from build123d import *
from OCP.BRepFilletAPI import BRepFilletAPI_MakeChamfer

# Parameters (mm, degrees)
SKETCH_1_W                = 265
SKETCH_1_H                = 125
EXTRUDE_1_DEPTH           = 85
SKETCH_2_W                = 330
SKETCH_2_H                = 125
EXTRUDE_2_DEPTH           = 20
SKETCH_3_W                = 150
SKETCH_3_H                = 125
CUT_EXTRUDE_1_DEPTH       = 5
SKETCH_4_R                = 40
CUT_EXTRUDE_2_DEPTH       = 206.319872394
SKETCH_5_W                = 210
SKETCH_5_H                = 125
CUT_EXTRUDE_3_DEPTH       = 80
CHAMFER_2_SIZE            = 56
CHAMFER_2_SIZE2           = 32.331615075
SKETCH_10_R               = 4.5
SKETCH_10_R_2             = 4
CUT_EXTRUDE_4_DEPTH       = 196.847517217
HOLE_WIZARD_M16_1_D       = 14
HOLE_WIZARD_M16_1_DEPTH   = 20
HOLE_WIZARD_M16_1_TIP     = 4.206024333
CHAMFER_3_SIZE            = 1
HOLE_WIZARD_1_D           = 9
HOLE_WIZARD_1_CBORE_D     = 15
HOLE_WIZARD_1_CBORE_DEPTH = 9
HOLE_WIZARD_M8_1_D        = 6.8
HOLE_WIZARD_M8_1_DEPTH    = 22.25
HOLE_WIZARD_M8_1_TIP      = 2.042926105
FILLET_1_R                = 8
FILLET_2_R                = 2


with BuildPart() as part:
    # 草图1 → 凸台-拉伸1 (new body)
    with BuildSketch(Plane.XY):
        Rectangle(SKETCH_1_W, SKETCH_1_H)
    extrude(amount=EXTRUDE_1_DEPTH)

    # 草图2 → 凸台-拉伸2 (add)
    with BuildSketch(Plane.XY.offset(85)):
        Rectangle(SKETCH_2_W, SKETCH_2_H)
    extrude(amount=EXTRUDE_2_DEPTH)

    # 草图3 → 切除-拉伸1 (cut)
    with BuildSketch(Plane(origin=(0, 0, 0), x_dir=(-1, 0, 0), z_dir=(0, 0, -1))):
        Rectangle(SKETCH_3_W, SKETCH_3_H)
    extrude(amount=-CUT_EXTRUDE_1_DEPTH, mode=Mode.SUBTRACT)

    # 草图4 → 切除-拉伸2 (cut, through all)
    with BuildSketch(Plane(origin=(0, 0, 0), x_dir=(-1, 0, 0), z_dir=(0, 0, -1))):
        Circle(SKETCH_4_R)
    extrude(amount=-CUT_EXTRUDE_2_DEPTH, mode=Mode.SUBTRACT)

    # 草图5 → 切除-拉伸3 (cut)
    with BuildSketch(Plane.XY.offset(105)):
        Rectangle(SKETCH_5_W, SKETCH_5_H)
    extrude(amount=-CUT_EXTRUDE_3_DEPTH, mode=Mode.SUBTRACT)

    # 倒角2: one chamfer whose edges measure the first distance from different faces: ONE call of the kernel's chamfer builder (chamfer() names one face for all edges)
    chamfer_2_edges_1 = [part.edges().sort_by_distance(p)[0] for p in [
        (165, -62.5, 95),
    ]]
    chamfer_2_side_1 = [part.faces().sort_by_distance(p)[0] for p in [
        (165, 0, 95),
    ]]
    chamfer_2_edges_2 = [part.edges().sort_by_distance(p)[0] for p in [
        (-165, -62.5, 95),
    ]]
    chamfer_2_side_2 = [part.faces().sort_by_distance(p)[0] for p in [
        (-165, 0, 95),
    ]]
    chamfer_2 = BRepFilletAPI_MakeChamfer(part.part.solid().wrapped)
    for e in chamfer_2_edges_1:
        chamfer_2.Add(CHAMFER_2_SIZE, CHAMFER_2_SIZE2, e.wrapped, chamfer_2_side_1[0].wrapped)  # the first distance lies on this face
    for e in chamfer_2_edges_2:
        chamfer_2.Add(CHAMFER_2_SIZE, CHAMFER_2_SIZE2, e.wrapped, chamfer_2_side_2[0].wrapped)  # the first distance lies on this face
    add(Compound.cast(chamfer_2.Shape()), mode=Mode.REPLACE)

    # 草图10 → 切除-拉伸4 (cut, through all)
    with BuildSketch(Plane(origin=(0, 0, 85), x_dir=(-1, 0, 0), z_dir=(0, 0, -1))):
        with Locations((-150, 47.5)):
            Circle(SKETCH_10_R)
        with Locations((-150, -2.5)):
            Circle(SKETCH_10_R)
        with Locations((-150, 22.5)):
            Circle(SKETCH_10_R_2)
    cut_extrude_4 = extrude(amount=-CUT_EXTRUDE_4_DEPTH, mode=Mode.SUBTRACT)

    # M16 螺纹孔1
    with Locations(Plane(origin=(0, 0, 0), x_dir=(-1, 0, 0), z_dir=(0, 0, -1))):
        with Locations((105, 0), (-105, 0)):
            Hole(HOLE_WIZARD_M16_1_D / 2, depth=HOLE_WIZARD_M16_1_DEPTH)
            with Locations((0, 0, -(HOLE_WIZARD_M16_1_DEPTH + HOLE_WIZARD_M16_1_TIP / 2))):  # 118° drill point
                Cone(0, HOLE_WIZARD_M16_1_D / 2, HOLE_WIZARD_M16_1_TIP, mode=Mode.SUBTRACT)

    # 镜向1: 切除-拉伸4 across plane
    add(cut_extrude_4.mirror(Plane.ZY), mode=Mode.SUBTRACT)

    # 倒角3
    chamfer_3_edges = [part.edges().sort_by_distance(p)[0] for p in [
        (-154, 22.5, 85),
        (154, 22.5, 85),
    ]]
    chamfer(chamfer_3_edges, length=CHAMFER_3_SIZE)

    # 打孔尺寸根据内六角圆柱头螺钉的类型1 (through all)
    with Locations(Plane(origin=(0, 0, 85), x_dir=(-1, 0, 0), z_dir=(0, 0, -1))):
        with Locations((150, -2.5), (150, 47.5), (-150, -2.5), (-150, 47.5)):
            CounterBoreHole(HOLE_WIZARD_1_D / 2, HOLE_WIZARD_1_CBORE_D / 2, HOLE_WIZARD_1_CBORE_DEPTH)

    # M8 螺纹孔1
    with Locations(Plane(origin=(132.5, 0, 0), x_dir=(0, 0, -1), z_dir=(1, 0, 0))):
        with Locations((-10, 25), (-30, 25), (-30, -25), (-10, -25)):
            Hole(HOLE_WIZARD_M8_1_D / 2, depth=HOLE_WIZARD_M8_1_DEPTH)
            with Locations((0, 0, -(HOLE_WIZARD_M8_1_DEPTH + HOLE_WIZARD_M8_1_TIP / 2))):  # 118° drill point
                Cone(0, HOLE_WIZARD_M8_1_D / 2, HOLE_WIZARD_M8_1_TIP, mode=Mode.SUBTRACT)

    # 圆角1
    fillet_1_edges = [part.edges().sort_by_distance(p)[0] for p in [
        (132.5, 0, 85),
        (-132.5, 0, 85),
        (105, 0, 25),
        (-105, 0, 25),
    ]]
    fillet(fillet_1_edges, radius=FILLET_1_R)

    # 圆角2
    fillet_2_edges = [part.edges().sort_by_distance(p)[0] for p in [
        (75, 0, 5),
        (-75, 0, 5),
    ]]
    fillet(fillet_2_edges, radius=FILLET_2_R)


solid = part.part
For this review, take the finished solid that the model builds, in its own axes (mm). A direction names the side the tool comes from. Give positions to 0.01 mm unless a question says otherwise; leave off trailing zeros. Loops run counter-clockwise (first coordinate to the right, second up) from the corner with the lowest first, then second, coordinate; pieces in that order, holes last. Notation, with made-up numbers: M -22,-21 L 7,-21 A20 cw 7,17 Z; hole C -2.75,15 d11. An arc over 180 degrees is marked long. Answer as a JSON object with one key per item and string values. Group by question number.
Q1. Mouldability with a two-part tool opening along X and no side actions: class faces 1 (the flat face through (132.5, -1, 38)), 2 (the flat face through (105, -1, 70)), 3 (the cylindrical face through (121.22, -26.3, 33.14)) as +X half, -X half, draft (parallel to the pull), parting line (faces both ways), or undercut.
Q2. Add section A-A on x = 150. Give the boundary of the cut face in (y, z), and give its area (3 significant figures).
Q3. Add section C-C on x = -62.5. Give the boundary of the cut face in (y, z).
Q4. Add section B-B on y = 47.5. Give the number of separate pieces and of enclosed holes in the cut face, and give its area (3 significant figures).
Q5. For probe 1 along Y at (x, z) = (123, 10); probe 2 along Z at (x, y) = (118, -25); probe 3 along Y at (x, z) = (0, 17.75), list the stretches that pass through material, from the lowest coordinate up. Write a range as [from, to].
Q6. Insertion check: P1, Ø4.5, axis at x = -152.5, y = 47, coming from the -Z side; P2, Ø6, axis at y = 25, z = 23, coming from the -X side; P3, Ø1, axis at y = -16.5, z = 59.5, coming from the +X side. Each pin has a flat end and moves straight along its axis. Give the tip position at first contact, or say it passes through.
Q7. Tool access review of faces 4 (the flat face through (155, 20, 85)), 5 (the flat face through (1, 43, 5)), 6 (the flat face through (-155, 48, 94)): name each direction out of +Z, -Z, +X, -X, +Y, -Y from which nothing blocks a thin tool from reaching the whole face with its end or side.
Checked values:
{
 "1": {"face 1": "+X half", "face 2": "undercut", "face 3": "draft"},
 "2": {"outline": "M -32.48,85 L -10,85 L -10,94 L -7,94 L -7,105 L -32.48,105 Z; M 2,94 L 5,94 L 5,85 L 17.5,85 L 18.5,86 L 18.5,105 L 2,105 Z; M 26.5,86 L 27.5,85 L 40,85 L 40,94 L 43,94 L 43,105 L 26.5,105 Z; M 52,94 L 55,94 L 55,85 L 62.5,85 L 62.5,105 L 52,105 Z", "area": "1,270 mm²"},
 "3": {"outline": "M -62.5,5 L 62.5,5 L 62.5,25 L -62.5,25 Z"},
 "4": {"separate pieces": "3", "enclosed holes": "0", "area": "11,200 mm²"},
 "5": {"probe 1": "[-62.5, -28.4], [-21.6, 21.6], [28.4, 62.5]", "probe 2": "[0, 6.6], [13.4, 26.6], [33.4, 105]", "probe 3": "[-62.5, -40], [40, 62.5]"},
 "6": {"P1": "z = 94", "P2": "x = -132.5", "P3": "x = 132.5"},
 "7": {"face 4": "-Z, +X, +Y, -Y", "face 5": "-Z, +Y, -Y", "face 6": "-Z"}
}
